```python
from build123d import *

# Parameters (mm, degrees)
ESQUISSE1_R                         = 6
BOSS_EXTRU_1_DEPTH                  = 4
CONG_1_R                            = 10
BOSS_EXTRU_2_REACH                  = 34.5
BOSS_EXTRU_2_DIRECTION_2_REACH      = 34.5
CONG_2_R                            = 2
ENL_V_MAT_EXTRU_1_REACH             = 6
ENL_V_MAT_EXTRU_1_DIRECTION_2_DEPTH = 5
DIAM_TRE_DU_PER_AGE_14_0_14_1_D     = 14


with BuildPart() as part:
    # Esquisse1 → Boss.-Extru.1 (new body)
    with BuildSketch(Plane.XY):
        Polygon((-32.5, -9.841659782), (-12.5, -34.841659782), (12.5, -34.841659782), (32.5, -9.841659782), (32.5, 25.158340218), (-32.5, 25.158340218), align=None)
        with Locations((-17.5, 12.158340218)):
            Circle(ESQUISSE1_R, mode=Mode.SUBTRACT)
        with Locations((17.5, 12.158340218)):
            Circle(ESQUISSE1_R, mode=Mode.SUBTRACT)
    extrude(amount=BOSS_EXTRU_1_DEPTH)

    # Congé1
    cong_1_edges = [part.edges().sort_by_distance(p)[0] for p in [
        (-32.5, 25.158340218, 2),
        (32.5, 25.158340218, 2),
        (32.5, -9.841659782, 2),
        (12.5, -34.841659782, 2),
        (-12.5, -34.841659782, 2),
        (-32.5, -9.841659782, 2),
    ]]
    fillet(cong_1_edges, radius=CONG_1_R)

    # Boss.-Extru.2: up to this face of the body (flat: up to its plane)
    boss_extru_2_end = Plane(part.part.faces().sort_by_distance((32.5, 4.412245514, 2))[0])
    # Esquisse2 → Boss.-Extru.2 (add, up to the picked face)
    with BuildSketch(Plane(origin=(0, 0, 0), x_dir=(0, 0, -1), z_dir=(1, 0, 0)), mode=Mode.PRIVATE) as boss_extru_2_sk1:
        with BuildLine():
            Line((0, 0), (24, 0))
            ThreePointArc((24, 0), (31.071067812, -2.928932188), (34, -10))
            Line((34, -10), (34, -35))
            Line((34, -35), (30, -35))
            Line((30, -35), (30, -10))
            ThreePointArc((30, -10), (28.242640687, -5.757359313), (24, -4))
            Line((24, -4), (0, -4))
            Line((0, -4), (0, 0))
        make_face()
    boss_extru_2_tool1 = split(extrude(boss_extru_2_sk1.sketch, amount=BOSS_EXTRU_2_REACH, mode=Mode.PRIVATE), bisect_by=boss_extru_2_end, keep=Keep.BOTH, mode=Mode.PRIVATE)
    add(boss_extru_2_tool1.solids().sort_by(Axis((0, -0.487955, -12), (1, 0, 0)))[0])

    # Boss.-Extru.2 direction 2: up to this face of the body (flat: up to its plane)
    boss_extru_2_direction_2_end = Plane(part.part.faces().sort_by_distance((-32.5, 4.412245514, 2))[0])
    # Esquisse2 → Boss.-Extru.2 direction 2 (add, up to the picked face)
    with BuildSketch(Plane(origin=(0, 0, 0), x_dir=(0, 0, -1), z_dir=(1, 0, 0)), mode=Mode.PRIVATE) as boss_extru_2_direction_2_sk1:
        with BuildLine():
            Line((0, 0), (24, 0))
            ThreePointArc((24, 0), (31.071067812, -2.928932188), (34, -10))
            Line((34, -10), (34, -35))
            Line((34, -35), (30, -35))
            Line((30, -35), (30, -10))
            ThreePointArc((30, -10), (28.242640687, -5.757359313), (24, -4))
            Line((24, -4), (0, -4))
            Line((0, -4), (0, 0))
        make_face()
    boss_extru_2_direction_2_tool1 = split(extrude(boss_extru_2_direction_2_sk1.sketch, amount=-BOSS_EXTRU_2_DIRECTION_2_REACH, mode=Mode.PRIVATE), bisect_by=boss_extru_2_direction_2_end, keep=Keep.BOTH, mode=Mode.PRIVATE)
    add(boss_extru_2_direction_2_tool1.solids().sort_by(Axis((0, -0.487955, -12), (-1, 0, 0)))[0])

    # Congé2
    cong_2_edges = [part.edges().sort_by_distance(p)[0] for p in [
        (0, 0, 0),
    ]]
    fillet(cong_2_edges, radius=CONG_2_R)

    # Esquisse3 → Enlèv. mat.-Extru.1 (cut, up to next)
    with BuildSketch(Plane.XY.offset(-30), mode=Mode.PRIVATE) as enl_v_mat_extru_1_sk1:
        with BuildLine():
            Line((-32.5, -6.333849189), (-38.653299958, -6.333849189))
            Line((-38.653299958, -6.333849189), (-39.385367291, -42.953606415))
            Line((-39.385367291, -42.953606415), (40.318463565, -42.953606415))
            Line((40.318463565, -42.953606415), (40.318463565, -6.333849189))
            Line((40.318463565, -6.333849189), (32.5, -6.333849189))
            ThreePointArc((32.5, -6.333849189), (31.936283192, -9.643918603), (30.308688094, -12.580799664))
            Line((30.308688094, -12.580799664), (15.50243962, -31.088610258))
            ThreePointArc((15.50243962, -31.088610258), (12.02563883, -33.854692146), (7.693751525, -34.841659782))
            Line((7.693751525, -34.841659782), (-7.693751525, -34.841659782))
            ThreePointArc((-7.693751525, -34.841659782), (-12.02563883, -33.854692146), (-15.50243962, -31.088610258))
            Line((-15.50243962, -31.088610258), (-30.308688094, -12.580799664))
            ThreePointArc((-30.308688094, -12.580799664), (-31.936283192, -9.643918603), (-32.5, -6.333849189))
        make_face()
    enl_v_mat_extru_1_tool1 = extrude(enl_v_mat_extru_1_sk1.sketch, amount=-ENL_V_MAT_EXTRU_1_REACH, mode=Mode.PRIVATE) & part.part
    add(enl_v_mat_extru_1_tool1.solids().sort_by_distance((-35.57665, -7.210987, -30))[0], mode=Mode.SUBTRACT)

    # Esquisse3 → Enlèv. mat.-Extru.1 direction 2 (cut)
    with BuildSketch(Plane.XY.offset(-30)):
        with BuildLine():
            Line((-32.5, -6.333849189), (-38.653299958, -6.333849189))
            Line((-38.653299958, -6.333849189), (-39.385367291, -42.953606415))
            Line((-39.385367291, -42.953606415), (40.318463565, -42.953606415))
            Line((40.318463565, -42.953606415), (40.318463565, -6.333849189))
            Line((40.318463565, -6.333849189), (32.5, -6.333849189))
            ThreePointArc((32.5, -6.333849189), (31.936283192, -9.643918603), (30.308688094, -12.580799664))
            Line((30.308688094, -12.580799664), (15.50243962, -31.088610258))
            ThreePointArc((15.50243962, -31.088610258), (12.02563883, -33.854692146), (7.693751525, -34.841659782))
            Line((7.693751525, -34.841659782), (-7.693751525, -34.841659782))
            ThreePointArc((-7.693751525, -34.841659782), (-12.02563883, -33.854692146), (-15.50243962, -31.088610258))
            Line((-15.50243962, -31.088610258), (-30.308688094, -12.580799664))
            ThreePointArc((-30.308688094, -12.580799664), (-31.936283192, -9.643918603), (-32.5, -6.333849189))
        make_face()
    extrude(amount=ENL_V_MAT_EXTRU_1_DIRECTION_2_DEPTH, mode=Mode.SUBTRACT)

    # Diamètre du perçage Ø14.0 (14)1 (through all)
    with Locations(Plane.XY.offset(4)):
        with Locations((0, -20.841659782)):
            Hole(DIAM_TRE_DU_PER_AGE_14_0_14_1_D / 2)


solid = part.part
```
Part model, mm, in its own coordinate system. A direction names the side the tool comes from. Round coordinates to 2 decimals unless told otherwise and drop trailing zeros. Order: outer loops, then holes, each group sorted by start corner. A loop starts at its lowest first (then second) coordinate and runs counter-clockwise, first axis right, second up. Notation, with made-up numbers: M 13.5,38.25 L 45.5,38.25 A17 ccw 45.5,51.25 Z; hole C 54,67 d2. An arc over 180 degrees is marked long. Answer in a Markdown table with one row per item. Add a question column.
Q1. Mould opens along Y. For faces 1 (the face through (0.45, 0.57, -0.6)), 2 (the face through (-22.802, -21.964, -31.972)), 3 (the face through (23.042, 9.86, 1.972)), 4 (the face through (1.517, -27.675, -32.028)) say: +Y half, -Y half, draft (parallel to the pull), parting line (faces both ways), or undercut.
Q2. Wall check: L1, parallel to Z at x = -23.5, y = -15.5; L2, parallel to Y at x = 12.5, z = -10; L3, parallel to Z at x = -2, y = 22. Give the ranges that are in metal, low to high. Write a range as from..to.
Q3. 3-axis set-ups, long thin cutter, end or side, ignore diameter. For faces 5 (the face through (0, 14, 0)), 6 (the face through (0.455, -5.804, -28.289)), 7 (the face through (29.5, 22.3, 2)): which of +Z, -Z, +X, -X, +Y, -Y reach the whole face in a straight line?
Q4. Cut at A-A on x = 0. Give the cut face in (y, z).
Q5. Cut at B-B on x = 17.5. Give the cut face in (y, z).
Q6. Cut at D-D on y = -15. Give the cut face in (x, z), and give its area (3 significant figures).
Q7. Cut at C-C on y = -29. Give the cut face in (x, z).
Q8. Pin check, flat tips, straight feed: pin 1 (4 mm diameter, centred on x = 9.5, z = -9, fed in from +Y); pin 2 (8.5 mm diameter, centred on x = 0, y = -20.84, fed in from +Z); pin 3 (11.5 mm diameter, centred on x = -13, y = 10, fed in from -Z); pin 4 (19 mm diameter, centred on x = -6, z = -15, fed in from -Y). Stop position of each tip, or through.
Established:
| question | item | result |
|---|---|---|
| 1 | face 1 | +Y half |
| 1 | face 2 | -Y half |
| 1 | face 3 | undercut |
| 1 | face 4 | undercut |
| 2 | L1 | z = -34..-30, 0..4 |
| 2 | L2 | y = -4..0 |
| 2 | L3 | z = 0..4 |
| 3 | face 5 | -Z, +X, -X, +Y |
| 3 | face 6 | +X, -X, -Y |
| 3 | face 7 | +Z, -Z, +X, +Y |
| 4 | outline | M -34.84,-34 L -27.84,-34 L -27.84,-30 L -34.84,-30 Z; M -34.84,0 L -27.84,0 L -27.84,4 L -34.84,4 Z; M -13.84,-34 L -10,-34 A10 ccw 0,-24 L 0,-2 A2 cw 2,0 L 25.16,0 L 25.16,4 L -13.84,4 L -13.84,0 L -4,0 L -4,-24 A6 cw -10,-30 L -13.84,-30 Z |
| 5 | outline | M -28.59,-34 L -10,-34 A10 ccw 0,-24 L 0,-2 A2 cw 2,0 L 6.16,0 L 6.16,4 L -28.59,4 L -28.59,0 L -4,0 L -4,-24 A6 cw -10,-30 L -28.59,-30 Z; M 18.16,0 L 25.16,0 L 25.16,4 L 18.16,4 Z |
| 6 | outline | M -28.37,-34 L -3.86,-34 L -3.86,-30 L -28.37,-30 Z; M -28.37,0 L -3.86,0 L -3.86,4 L -28.37,4 Z; M 3.86,-34 L 28.37,-34 L 28.37,-30 L 3.86,-30 Z; M 3.86,0 L 28.37,0 L 28.37,4 L 3.86,4 Z |
| 6 | area | 392 mm2 |
| 7 | outline | M -17.17,-34 L 17.17,-34 L 17.17,-30 L -17.17,-30 Z; M -17.17,0 L 17.17,0 L 17.17,4 L -17.17,4 Z |
| 8 | pin 1 | stops at y = 0 |
| 8 | pin 2 | passes through |
| 8 | pin 3 | stops at z = 0 |
| 8 | pin 4 | stops at y = -4.02 |
